Autodesk Fusion 360 part; units mm, degrees
sketch "Sketch1" plane through (0, 0, 0) normal (0, 0, 1) x (1, 0, 0)
  line L0 (2.4, 4.9) -> (-2.4, 4.9)
  line L1 (-2.4, 4.9) -> (-2.4, -4.9)
  line L2 (-2.4, -4.9) -> (2.4, -4.9)
  line L3 (2.4, -4.9) -> (2.4, 4.9)
  line L4 (2.4, 4.9) -> (-2.4, -4.9) construction
  line L5 (-2.4, 4.9) -> (2.4, -4.9) construction
  dimension "d1" = 4.8
  dimension "d2" = 9.8
extrude "Extrude1" add sketch "Sketch1" along normal blind 5
sketch "Sketch2" plane through (0, 0, 5) normal (0, 0, 1) x (1, 0, 0)
  line L0 (2.4, -4.9) -> (2.4, 4.9)
  line L1 (2.4, 4.9) -> (-2.4, 4.9)
  line L2 (-2.4, 4.9) -> (-2.4, -4.9)
  line L3 (-2.4, -4.9) -> (2.4, -4.9)
  circle A0 centre (0, 0) radius 10
  dimension "d5" = 20
extrude "Extrude2" add sketch "Sketch2" along normal blind 5 contours L0 L1 L2 L3 | A0
sketch "Sketch3" plane through (0, 0, 10) normal (0, 0, 1) x (1, 0, 0)
  circle A0 centre (0, 0) radius 10
  line L0 (-1.5, 2.75) -> (1.5, 2.75)
  line L1 (1.5, 2.75) -> (1.5, -2.75)
  line L2 (1.5, -2.75) -> (-1.5, -2.75)
  line L3 (-1.5, -2.75) -> (-1.5, 2.75)
  line L4 (-1.5, 2.75) -> (1.5, -2.75) construction
  line L5 (1.5, 2.75) -> (-1.5, -2.75) construction
  circle A1 centre (0, 0) radius 5
  dimension "d8" = 5.5
  dimension "d9" = 3
  dimension "d10" = 10
extrude "Extrude3" add sketch "Sketch3" along normal blind 6 contours A1
extrude "Extrude4" cut sketch "Sketch3" against normal blind 3 contours L0 L1 L2 L3
Geometry: final body of the model. Coordinates: model frame, mm. A direction names the side the tool comes from. Round coordinates to 2 decimals unless told otherwise and drop trailing zeros. Order: outer loops, then holes, each group sorted by start corner. A loop starts at its lowest first (then second) coordinate and runs counter-clockwise, first axis right, second up.
Q1. Section C-C, the plane y = 0. Output: boundary loops of the cut face in (x, z).
Result sheet:
outline: (-10, 5) - (-2.4, 5) - (-2.4, 0) - (2.4, 0) - (2.4, 5) - (10, 5) - (10, 10) - (5, 10) - (5, 16) - (1.5, 16) - (1.5, 7) - (-1.5, 7) - (-1.5, 16) - (-5, 16) - (-5, 10) - (-10, 10) - close
Q2. Pin query (flat end, axial travel): pin 1 (6 mm diameter, centred on x = -3.5, z = 12, fed in from +Y); pin 2 (3 mm diameter, centred on x = -3, y = -6.5, fed in from -Z); pin 3 (2 mm diameter, centred on y = -3, z = 2.5, fed in from +X). Return the tip coordinate at first contact, or that it passes through.
Result sheet:
pin 1: stops at y = 9.92
pin 2: stops at z = 5
pin 3: stops at x = 2.4
Q3. Material intervals for probe 1 along X at (y, z) = (-4.25, 3.5); probe 2 along Z at (x, y) = (8, -1); probe 3 along Y at (x, z) = (-0.5, 9), sorted ascending.
Result sheet:
probe 1: x = -2.4 to 2.4
probe 2: z = 5 to 10
probe 3: y = -9.99 to -2.75, 2.75 to 9.99
Q4. Mould query, pull axis X, two halves, no side actions, for faces 5 (the face through (0, 2.75, 11)), 6 (the face through (-1.08, 4.88, 12.96)), 7 (the face through (-2.4, 0, 2)). Classes: released by +X, released by -X, zero draft, split by the parting line, or undercut.
Result sheet:
face 5: undercut
face 6: split by the parting line
face 7: released by -X
Q5. Section B-B, the plane x = 0. Output: boundary loops of the cut face in (y, z).
Result sheet:
outline: (-10, 5) - (-4.9, 5) - (-4.9, 0) - (4.9, 0) - (4.9, 5) - (10, 5) - (10, 10) - (5, 10) - (5, 16) - (2.75, 16) - (2.75, 7) - (-2.75, 7) - (-2.75, 16) - (-5, 16) - (-5, 10) - (-10, 10) - close
Q6. Section D-D, the plane z = 5.5. Output: boundary loops of the cut face in (x, y).
Result sheet:
outline: circle Ø20 at (0, 0)
Q7. Section A-A, the plane z = 8. Output: boundary loops of the cut face in (x, y).
Result sheet:
outline: circle Ø20 at (0, 0); hole (-1.5, -2.75) - (1.5, -2.75) - (1.5, 2.75) - (-1.5, 2.75) - close
Q8. Access query for faces 1 (the face through (2.4, 0, 2)), 2 (the face through (0, 0, 7)), 3 (the face through (0, 4.9, 2)), 4 (the face through (0, -4.9, 2)). Directions: +Z, -Z, +X, -X, +Y, -Y. A direction counts if a zero-diameter tool reaches every point of the face in a straight line with its end or side. Return the directions, or none.
Result sheet:
face 1: -Z, +X, +Y, -Y
face 2: +Z
face 3: -Z, +X, -X, +Y
face 4: -Z, +X, -X, -Y
